```python
from build123d import *

# Parameters (mm, degrees)
CYLINDER001_R     = 2.5
CYLINDER001_DEPTH = 10
CYLINDER003_R     = 11.9
CYLINDER003_DEPTH = 16
CYLINDER002_R     = 2.5
CYLINDER002_DEPTH = 10
CYLINDER_R        = 14
CYLINDER_DEPTH    = 17
BOX_W             = 65
BOX_H             = 3
BOX_DEPTH         = 17
BOX001_W          = 65
BOX001_H          = 4
BOX001_DEPTH      = 11
BOX002_W          = 28
BOX002_H          = 13
BOX002_DEPTH      = 17
FILLET_R          = 5


with BuildPart() as cylinder001:
    # Cylinder001 → Cylinder001 (new body)
    with BuildSketch(Plane(origin=(-23.5, -14, 8.5), x_dir=(1, 0, 0), z_dir=(0, 1, 0))):
        Circle(CYLINDER001_R)
    extrude(amount=CYLINDER001_DEPTH)


with BuildPart() as cylinder003:
    # Cylinder003 → Cylinder003 (new body)
    with BuildSketch(Plane.XY.offset(1)):
        Circle(CYLINDER003_R)
    extrude(amount=CYLINDER003_DEPTH)


with BuildPart() as cone:
    # Cone → Cone (revolve)
    with BuildSketch(Plane(origin=(23.5, -11.5, 8.5), x_dir=(1, 0, 0), z_dir=(0, 0, 1))):
        Polygon((0, 0), (4.5, 2), (0, 2), align=None)
    revolve(axis=Axis((23.5, -11.5, 8.5), (0, 1, 0)))


with BuildPart() as cone001:
    # Cone001 → Cone001 (revolve)
    with BuildSketch(Plane(origin=(-23.5, -11.5, 8.5), x_dir=(1, 0, 0), z_dir=(0, 0, 1))):
        Polygon((0, 0), (4.5, 2), (0, 2), align=None)
    revolve(axis=Axis((-23.5, -11.5, 8.5), (0, 1, 0)))


with BuildPart() as fusion:
    # Cylinder002 → Cylinder002 (new body)
    with BuildSketch(Plane(origin=(23.5, -14, 8.5), x_dir=(1, 0, 0), z_dir=(0, 1, 0))):
        Circle(CYLINDER002_R)
    extrude(amount=CYLINDER002_DEPTH)

    # Fusion: union Cylinder001, Cylinder003, Cone, Cone001
    add(cylinder001.part)
    add(cylinder003.part)
    add(cone.part)
    add(cone001.part)


with BuildPart() as cylinder:
    # Cylinder → Cylinder (new body)
    with BuildSketch(Plane.XY):
        Circle(CYLINDER_R)
    extrude(amount=CYLINDER_DEPTH)


with BuildPart() as box:
    # Box → Box (new body)
    with BuildSketch(Plane(origin=(-32.5, -14, 0), x_dir=(1, 0, 0), z_dir=(0, 0, 1))):
        with Locations((32.5, 1.5)):
            Rectangle(BOX_W, BOX_H)
    extrude(amount=BOX_DEPTH)


with BuildPart() as box001:
    # Box001 → Box001 (new body)
    with BuildSketch(Plane(origin=(-32.5, -13.5, 3), x_dir=(1, 0, 0), z_dir=(0, 0, 1))):
        with Locations((32.5, 2)):
            Rectangle(BOX001_W, BOX001_H)
    extrude(amount=BOX001_DEPTH)


with BuildPart() as fillet_body:
    # Box002 → Box002 (new body)
    with BuildSketch(Plane(origin=(-14, -13, 0), x_dir=(1, 0, 0), z_dir=(0, 0, 1))):
        with Locations((14, 6.5)):
            Rectangle(BOX002_W, BOX002_H)
    extrude(amount=BOX002_DEPTH)

    # Fusion001: union Cylinder, Box, Box001
    add(cylinder.part)
    add(box.part)
    add(box001.part)

    # Cut: cut Fusion
    add(fusion.part, mode=Mode.SUBTRACT)

    # Fillet
    fillet_edges = [fillet_body.edges().sort_by_distance(p)[0] for p in [
        (32.5, -10.25, 3),
        (32.5, -10.25, 14),
        (-32.5, -10.25, 14),
        (-32.5, -10.25, 3),
    ]]
    fillet(fillet_edges, radius=FILLET_R)


solid = fillet_body.part
```
Design review of the part built by this model. Coordinates are the model's own, in mm. A direction names the side the tool comes from. Coordinates: 2 decimals unless noted, no trailing zeros. Order: outer loops, then holes, each group sorted by start corner. A loop starts at its lowest first (then second) coordinate and runs counter-clockwise, first axis right, second up. Notation, with made-up numbers: M -33,1.25 L 0,1.25 A9 ccw 0,9.25 Z; hole C 67.5,-25.75 d1. An arc over 180 degrees is marked long. Answer as a JSON object with one key per item and string values. Group by question number.
1) Add section C-C, the plane x = 5.5. Write out the cut boundary in (y, z).
2) Add section B-B, the plane y = -6.25. Write out the cut boundary in (x, z).
3) Mouldability with a two-part tool opening along Y and no side actions: class faces 1 (the cylindrical face through (-8.771, 8.043, 8.888)), 2 (the flat face through (-23, -11, 1)), 3 (the flat face through (-21, -10, 3)) as pulls with the +Y half, pulls with the -Y half, needs draft (parallel to the pull), parting line crosses it, or undercut.
4) Tool access review of faces 4 (the cylindrical face through (31.07, -10.24, 4.5)), 5 (the cylindrical face through (-31.07, -10.24, 12.5)), 6 (the flat face through (21, -10, 14)): name each direction out of +Z, -Z, +X, -X, +Y, -Y from which nothing blocks a thin tool from reaching the whole face with its end or side.
5) Wall thickness on L1, parallel to X at y = -12.3, z = 8.5; L2, parallel to Z at x = 23.5, y = -12.65; L3, parallel to Y at x = 0, z = 8.75: over which ranges is each line inside the solid? List them lowest first.
6) For pin 1 (1.5 mm diameter, centred on y = -1.5, z = 14.5, fed in from -X); pin 2 (5 mm diameter, centred on y = -3, z = 10.5, fed in from +X); pin 3 (9 mm diameter, centred on y = -6, z = 5, fed in from +X), all flat-tipped, find the tip position at first contact; note any pin that passes through.
7) Add section A-A, the plane x = -23.5. Write out the cut boundary in (y, z), then the cut area to 3 significant figures.
Computed values:
{
 "1": {"outline": "M -14,0 L 12.87,0 L 12.87,17 L 10.55,17 L 10.55,1 L -10.55,1 L -10.55,17 L -14,17 Z"},
 "2": {"outline": "M -14,0 L 14,0 L 14,17 L 10.13,17 L 10.13,1 L -10.13,1 L -10.13,17 L -14,17 Z"},
 "3": {"face 1": "undercut", "face 2": "pulls with the +Y half", "face 3": "needs draft"},
 "4": {"face 4": "-Z, +X, +Y", "face 5": "+Z, -X, +Y", "face 6": "+Z, +X, +Y"},
 "5": {"L1": "x = -32.5 to -26, -21 to 21, 26 to 32.5", "L2": "z = 0 to 6, 11 to 17", "L3": "y = -14 to -11.9, 11.9 to 14"},
 "6": {"pin 1": "stops at x = -14", "pin 2": "stops at x = 14", "pin 3": "stops at x = 32.5"},
 "7": {"outline": "M -14,0 L -11,0 L -11,3 L -9.5,3 L -9.5,4 L -10.39,6 L -14,6 Z; M -14,11 L -10.39,11 L -9.5,13 L -9.5,14 L -11,14 L -11,17 L -14,17 Z", "area": "43.2 mm^2"}
}
